Could you check a few things on this model? Use its own coordinates, in mm. Face numbers are marked on the shaded views. A direction names the side the tool comes from. Round coordinates to 2 decimals unless told otherwise and drop trailing zeros. Loops run counter-clockwise (first coordinate to the right, second up) from the corner with the lowest first, then second, coordinate; pieces in that order, holes last. Notation, with made-up numbers: (6, -33) -> (15, -33) arc R10 ccw to (15, -18) -> close; hole circle Ø8 at (66, -38). An arc over 180 degrees is marked (long way). Write each question's results on one line, items separated by ' | '.
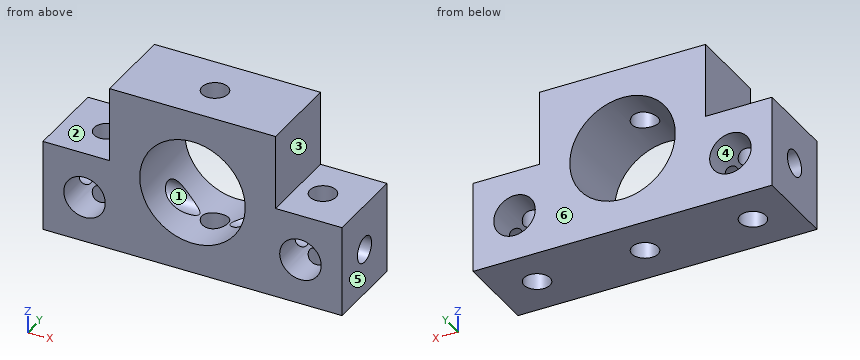
from build123d import *

# Parameters (mm, degrees)
SKETCH1_W                  = 18
SKETCH1_H                  = 10
BOSS_EXTRUDE1_DEPTH        = 5
SKETCH2_W                  = 4
SKETCH2_H                  = 4.5
CUT_EXTRUDE1_DEPTH         = 15.352700094
SKETCH3_W                  = 4
SKETCH3_H                  = 4.5
CUT_EXTRUDE2_DEPTH         = 15.352700094
F_2_5_2_5_DIAMETER_HOLE1_D = 2.5
HOLE1_D                    = 1.567
HOLE1_DEPTH                = 19.526024769
HOLE2_D                    = 1.567
HOLE2_DEPTH                = 7.276024769
HOLE3_D                    = 6.35
HOLE4_D                    = 1.567
HOLE4_DEPTH                = 11.923191142


with BuildPart() as part:
    # Sketch1 → Boss-Extrude1 (new body)
    with BuildSketch(Plane.XZ.offset(5)):
        with Locations((0, 5)):
            Rectangle(SKETCH1_W, SKETCH1_H)
    extrude(amount=-BOSS_EXTRUDE1_DEPTH)

    # Sketch2 → Cut-Extrude1 (cut, through all)
    with BuildSketch(Plane(origin=(0, 0, 0), x_dir=(-1, 0, 0), z_dir=(0, 1, 0))):
        with Locations((7, 7.75)):
            Rectangle(SKETCH2_W, SKETCH2_H)
    extrude(amount=-CUT_EXTRUDE1_DEPTH, mode=Mode.SUBTRACT)

    # Sketch3 → Cut-Extrude2 (cut, through all)
    with BuildSketch(Plane(origin=(0, 0, 0), x_dir=(-1, 0, 0), z_dir=(0, 1, 0))):
        with Locations((-7, 7.75)):
            Rectangle(SKETCH3_W, SKETCH3_H)
    extrude(amount=-CUT_EXTRUDE2_DEPTH, mode=Mode.SUBTRACT)

    # Ø2.5 (2.5) Diameter Hole1 (through all)
    with Locations(Plane(origin=(0, 0, 0), x_dir=(1, 0, 0), z_dir=(0, 1, 0))):
        with Locations((6.5, -2.75), (-6.5, -2.75)):
            Hole(F_2_5_2_5_DIAMETER_HOLE1_D / 2)

    # Hole1
    with Locations(Plane(origin=(9, 0, 0), x_dir=(0, 0, -1), z_dir=(1, 0, 0))):
        with Locations((-2.75, -2.5)):
            Hole(HOLE1_D / 2, depth=HOLE1_DEPTH)

    # Hole2
    with Locations(Plane.XY.offset(5.5)):
        with Locations((6.5, -2.5), (-6.5, -2.5)):
            Hole(HOLE2_D / 2, depth=HOLE2_DEPTH)

    # Hole3 (through all)
    with Locations(Plane(origin=(0, 0, 0), x_dir=(1, 0, 0), z_dir=(0, 1, 0))):
        with Locations((0, -5)):
            Hole(HOLE3_D / 2)

    # Hole4
    with Locations(Plane.XY.offset(10)):
        with Locations((0, -2.5)):
            Hole(HOLE4_D / 2, depth=HOLE4_DEPTH)


solid = part.part
1) I need wall thicknesses on line 1 (X direction, y = -2.5, z = 0.7); line 2 (Y direction, x = 6.5, z = 4.7); line 3 (X direction, y = -4.6, z = 2.5). Which ranges of each line are inside material? Lowest first, please.
Model answer:
line 1: x = -9 to -7.28, -5.72 to -0.78, 0.78 to 5.72, 7.28 to 9 | line 2: y = -5 to -3.28, -1.72 to 0 | line 3: x = -9 to -7.72, -5.28 to -1.96, 1.96 to 5.28, 7.72 to 9
2) For the marked faces 1, 2 and 3, which set-ups out of +Z, -Z, +X, -X, +Y, -Y let a thin tool reach every point of the face, with its end or its side?
Model answer:
face 1: +X, -X | face 2: +Z, -X, +Y, -Y | face 3: +Z, +X, +Y, -Y
3) I want a section at C-C, the plane y = -1.35. Write out the boundary of the cut face in (x, z) (3 decimals).
Model answer:
outline: (-9, 0) -> (9, 0) -> (9, 5.5) -> (5, 5.5) -> (5, 10) -> (-5, 10) -> (-5, 5.5) -> (-9, 5.5) -> close; hole circle Ø2.5 at (-6.5, 2.75); hole circle Ø6.35 at (0, 5); hole circle Ø2.5 at (6.5, 2.75)
4) I want a section at B-B, the plane z = 9. Write out the boundary of the cut face in (x, y).
Model answer:
outline: (-5, -5) -> (5, -5) -> (5, 0) -> (-5, 0) -> close; hole circle Ø1.57 at (0, -2.5)
5) I want a section at A-A, the plane x = 0. Write out the boundary of the cut face in (y, z) (1 decimal), plus the area to 3 significant figures.
Model answer:
outline: (-5, 0) -> (-3.3, 0) -> (-3.3, 1.8) -> (-5, 1.8) -> close; (-5, 8.2) -> (-3.3, 8.2) -> (-3.3, 10) -> (-5, 10) -> close; (-1.7, 0) -> (0, 0) -> (0, 1.8) -> (-1.7, 1.8) -> close; (-1.7, 8.2) -> (0, 8.2) -> (0, 10) -> (-1.7, 10) -> close | area: 12.5 mm2
6) I'm going to push flat-ended pins straight in: pin 1 (1.3 mm diameter, centred on y = -1.5, z = 9, fed in from +X); pin 2 (2 mm diameter, centred on x = -6.5, y = -2.5, fed in from +Z); pin 3 (2 mm diameter, centred on y = -1.5, z = 7, fed in from -X). Where does each tip first touch, or does it pass through?
Model answer:
pin 1: stops at x = 5 | pin 2: stops at z = 5.5 | pin 3: stops at x = -5
7) If we mould it in two halves opening along X, with no side actions, what happens to the marked faces 4, 5 and 6? For each: released by +X, released by -X, zero draft, split by the parting line, or undercut.
Model answer:
face 4: undercut | face 5: released by +X | face 6: zero draft
8) I want a section at D-D, the plane z = 7.25. Write out the boundary of the cut face in (x, y).
Model answer:
outline: (-5, -5) -> (-2.24, -5) -> (-2.24, 0) -> (-5, 0) -> close; (2.24, -5) -> (5, -5) -> (5, 0) -> (2.24, 0) -> close
